from build123d import *

# Parameters (mm, degrees)
SKETCH1_W                        = 21.336
SKETCH1_H                        = 5.08
BOSS_EXTRUDE1_DEPTH              = 2.54
FILLET1_R                        = 1.27
SKETCH8_W                        = 3.556
SKETCH8_H                        = 2.54
CUT_EXTRUDE1_DEPTH               = 2.54
F_97_0_0059_DIAMETER_HOLE1_D     = 1.651
F_97_0_0059_DIAMETER_HOLE1_DEPTH = 1.524
F_97_0_0059_DIAMETER_HOLE1_TIP   = 0.496010441
F_0_80_TAPPED_HOLE1_D            = 1.19126
F_0_80_TAPPED_HOLE1_DEPTH        = 4.064
F_0_80_TAPPED_HOLE1_TIP          = 0.357890611


with BuildPart() as part:
    # Sketch1 → Boss-Extrude1 (new body)
    with BuildSketch(Plane(origin=(0, 0, 0), x_dir=(1, 0, 0), z_dir=(0, 1, 0))):
        with Locations((1.778, 2.54)):
            Rectangle(SKETCH1_W, SKETCH1_H)
    extrude(amount=BOSS_EXTRUDE1_DEPTH)

    # Fillet1
    fillet1_edges = [part.edges().sort_by_distance(p)[0] for p in [
        (-8.89, 0, -2.54),
        (-8.89, 2.54, -2.54),
        (12.446, 0, -2.54),
        (12.446, 2.54, -2.54),
    ]]
    fillet(fillet1_edges, radius=FILLET1_R - 0.0001)  # a hair under: the kernel refuses the full size

    # Sketch8 → Cut-Extrude1 (cut)
    with BuildSketch(Plane(origin=(0, 2.54, 0), x_dir=(1, 0, 0), z_dir=(0, 1, 0))):
        with Locations((10.668, 2.596814381)):
            Rectangle(SKETCH8_W, SKETCH8_H)
    extrude(amount=-CUT_EXTRUDE1_DEPTH, mode=Mode.SUBTRACT)

    # #97 (0.0059) Diameter Hole1
    with Locations(Plane.XY):
        with Locations((11.176, 1.27)):
            Hole(F_97_0_0059_DIAMETER_HOLE1_D / 2, depth=F_97_0_0059_DIAMETER_HOLE1_DEPTH)
            with Locations((0, 0, -(F_97_0_0059_DIAMETER_HOLE1_DEPTH + F_97_0_0059_DIAMETER_HOLE1_TIP / 2))):  # 118° drill point
                Cone(0, F_97_0_0059_DIAMETER_HOLE1_D / 2, F_97_0_0059_DIAMETER_HOLE1_TIP, mode=Mode.SUBTRACT)

    # #0-80 Tapped Hole1
    with Locations(Plane.XY.offset(-3.866814381)):
        with Locations((11.176, 1.27)):
            Hole(F_0_80_TAPPED_HOLE1_D / 2, depth=F_0_80_TAPPED_HOLE1_DEPTH)
            with Locations((0, 0, -(F_0_80_TAPPED_HOLE1_DEPTH + F_0_80_TAPPED_HOLE1_TIP / 2))):  # 118° drill point
                Cone(0, F_0_80_TAPPED_HOLE1_D / 2, F_0_80_TAPPED_HOLE1_TIP, mode=Mode.SUBTRACT)


solid = part.part
Source: CAD feature listing. Evaluate the final solid. Frame: model axes, mm. A direction names the side the tool comes from. Give positions to 0.01 mm unless a question says otherwise; leave off trailing zeros. Write item = value, one per line. Start each with the question number.
Q1. Reachability of faces 1 (the cylindrical face through (10.413, 0.954, -0.673)), 2 (the flat face through (2, 2.54, -3)), 3 (the flat face through (10, 1, -1.327)) from +Z, -Z, +X, -X, +Y, -Y: full face, straight path, thin tool, end or side. Return the list, or none.
Q2. Draft query along X for faces 4 (the cylindrical face through (12.08, 2.16, -0.67)), 5 (the cylindrical face through (11.62, 1.67, -4.48)), 6 (the cylindrical face through (-8.528, 0.382, -2.576)). Return one class per face: +X half, -X half, draft (parallel to the pull), parting line (faces both ways), or undercut.
Q3. Material intervals for probe 1 along Z at (x, y) = (9.5, 1.3); probe 2 along X at (y, z) = (1.2, -4.65); probe 3 along X at (y, z) = (1.85, -3.7), sorted ascending.
Computed values:
q1.face_1 = +Z
q1.face_2 = +Z, -Z, +X, -X, +Y
q1.face_3 = +X, +Y, -Y
q2.face_4 = +X half
q2.face_5 = undercut
q2.face_6 = -X half
q3.probe_1 = -5.08 to -3.87, -1.33 to 0
q3.probe_2 = -8.89 to 10.58, 11.77 to 12.44
q3.probe_3 = -8.75 to 8.89
